Design review of the part built by this model. Coordinates are the model's own, in mm. Face numbers are marked on the shaded views. Coordinates: 2 decimals unless noted, no trailing zeros. Loops run counter-clockwise (first coordinate to the right, second up) from the corner with the lowest first, then second, coordinate; pieces in that order, holes last. Notation, with made-up numbers: (88, -18) - (110, -18) arc R18 cw to (110, 0) - close; hole circle Ø11 at (0, 7.5). An arc over 180 degrees is marked (long way). Answer in a Markdown table with one row per item. Add a question column.
(1) We need section A-A, the plane x = 3.8. Write out the cut boundary in (y, z).
(2) Clearance check with flat-ended pins moving along their axes: pin 1 (12 mm diameter, centred on y = -18, z = 90, fed in from +X); pin 2 (5 mm diameter, centred on y = -19.5, z = 28, fed in from +X); pin 3 (5 mm diameter, centred on x = 12.5, z = 86.5, fed in from -Y). State where each tip first meets the part, or that it passes through.
(3) We need section D-D, the plane x = 59.9. Write out the cut boundary in (y, z), plus the area to 3 significant figures.
(4) To check wall thickness, follow L1, parallel to Z at x = 116, y = -1.8; L2, parallel to X at y = -1.65, z = 115.9; L3, parallel to X at y = -2, z = 27. State the ranges of each line that lie inside material, in increasing order. Write a range as [from, to].
(5) We need section C-C, the plane z = 59.8. Write out the cut boundary in (x, y), plus the area to 3 significant figures.
(6) We need section B-B, the plane z = 3.7. Write out the cut boundary in (x, y), plus the area to 3 significant figures.
(7) The part is to be moulded in two halves that separate along X. For the marked faces 1 and 2, say which applies: released by +X, released by -X, zero draft, split by the parting line, or undercut.
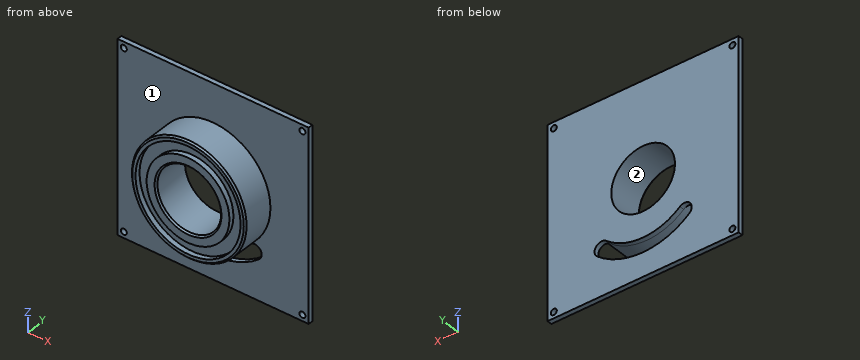
from build123d import *

# Parameters (mm, degrees)
SKETCH054_W     = 120
SKETCH054_H     = 120
PAD015_DEPTH    = 3
SKETCH065_R     = 1.9
POCKET034_DEPTH = 3.001
SKETCH064_R     = 20
POCKET036_DEPTH = 3.001
SKETCH058_R     = 36
PAD013_DEPTH    = 20
SKETCH055_R     = 20
POCKET035_DEPTH = 20.001
SKETCH056_R     = 33
SKETCH056_R_2   = 26
POCKET037_DEPTH = 3.2
CHAMFER003_SIZE = 1
CHAMFER002_SIZE = 1
POCKET042_DEPTH = 3.001


with BuildPart() as part:
    # Sketch054 → Pad015 (new body)
    with BuildSketch(Plane.XZ):
        with Locations((60, 60)):
            Rectangle(SKETCH054_W, SKETCH054_H)
    extrude(amount=PAD015_DEPTH)

    # Sketch065 (on Face6 of Pad015) → Pocket034 (cut, through all)
    with BuildSketch(Plane.XZ.offset(3)):
        with Locations((3.9, 3.9)):
            Circle(SKETCH065_R)
        with Locations((116.1, 3.9)):
            Circle(SKETCH065_R)
        with Locations((116.1, 116.1)):
            Circle(SKETCH065_R)
        with Locations((3.9, 116.1)):
            Circle(SKETCH065_R)
    extrude(amount=-POCKET034_DEPTH, mode=Mode.SUBTRACT)

    # Sketch064 (on Face5 of Pocket034) → Pocket036 (cut, through all)
    with BuildSketch(Plane.XZ.offset(3)):
        with Locations((60, 60)):
            Circle(SKETCH064_R)
    extrude(amount=-POCKET036_DEPTH, mode=Mode.SUBTRACT)

    # Sketch058 (on Face5 of Pocket036) → Pad013 (join)
    with BuildSketch(Plane.XZ.offset(3)):
        with Locations((60, 60)):
            Circle(SKETCH058_R)
    extrude(amount=PAD013_DEPTH)

    # Sketch055 (on Face13 of Pad013) → Pocket035 (cut, through all)
    with BuildSketch(Plane(origin=(0, -3, 0), x_dir=(1, 0, 0), z_dir=(0, 1, 0))):
        with Locations((60, -60)):
            Circle(SKETCH055_R)
    extrude(amount=-POCKET035_DEPTH, mode=Mode.SUBTRACT)

    # Sketch056 (on Face14 of Pocket035) → Pocket037 (cut)
    with BuildSketch(Plane.XZ.offset(23)):
        with Locations((60, 60)):
            Circle(SKETCH056_R)
        with Locations((60, 60)):
            Circle(SKETCH056_R_2, mode=Mode.SUBTRACT)
    extrude(amount=-POCKET037_DEPTH, mode=Mode.SUBTRACT)

    # Chamfer003
    chamfer003_edges = [part.edges().sort_by_distance(p)[0] for p in [
        (40, -23, 60),
    ]]
    chamfer(chamfer003_edges, length=CHAMFER003_SIZE)

    # Chamfer002
    chamfer002_edges = [part.edges().sort_by_distance(p)[0] for p in [
        (24, -23, 60),
    ]]
    chamfer(chamfer002_edges, length=CHAMFER002_SIZE)

    # Sketch066 (on Face3 of Chamfer002) → Pocket042 (cut, through all)
    with BuildSketch(Plane.XZ.offset(3)):
        with BuildLine():
            ThreePointArc((36.859646, 32.4224), (60, 24), (83.140354, 32.4224))
            ThreePointArc((88.925456, 25.528011), (89.480105, 31.867761), (83.140354, 32.4224))
            ThreePointArc((31.074571, 25.527989), (60.000017, 15), (88.925456, 25.528011))
            ThreePointArc((36.859646, 32.4224), (30.519908, 31.867728), (31.074571, 25.527989))
        make_face()
    extrude(amount=-POCKET042_DEPTH, mode=Mode.SUBTRACT)


with BuildPart() as part_1:
    # Body007 placement: moved
    add(part.part.moved(Location((-0.1, 0.5, -0.2))))


solid = part_1.part
Responses:
| question | item | result |
|---|---|---|
| 1 | outline | (-2.5, -0.2) - (0.5, -0.2) - (0.5, 1.8) - (-2.5, 1.8) - close; (-2.5, 5.6) - (0.5, 5.6) - (0.5, 114) - (-2.5, 114) - close; (-2.5, 117.8) - (0.5, 117.8) - (0.5, 119.8) - (-2.5, 119.8) - close |
| 2 | pin 1 | stops at x = 86.55 |
| 2 | pin 2 | stops at x = 80.82 |
| 2 | pin 3 | stops at y = -2.5 |
| 3 | outline | (-22.5, 24.8) - (-21.5, 23.8) - (0.5, 23.8) - (0.5, 39.8) - (-21.5, 39.8) - (-22.5, 38.8) - (-22.5, 33.8) - (-19.3, 33.8) - (-19.3, 26.8) - (-22.5, 26.8) - close; (-22.5, 80.8) - (-21.5, 79.8) - (0.5, 79.8) - (0.5, 119.8) - (-2.5, 119.8) - (-2.5, 95.8) - (-21.5, 95.8) - (-22.5, 94.8) - (-22.5, 92.8) - (-19.3, 92.8) - (-19.3, 85.8) - (-22.5, 85.8) - close; (-2.5, -0.2) - (0.5, -0.2) - (0.5, 14.8) - (-2.5, 14.8) - close |
| 3 | area | 806 mm2 |
| 4 | L1 | z = [-0.2, 1.8], [5.6, 114], [117.8, 119.8] |
| 4 | L2 | x = [-0.1, 1.9], [5.7, 114.1], [117.9, 119.9] |
| 4 | L3 | x = [-0.1, 29.73], [45.06, 74.74], [90.07, 119.9] |
| 5 | outline | (-0.1, -2.5) - (23.9, -2.5) - (23.9, -21.5) - (24.9, -22.5) - (26.9, -22.5) - (26.9, -19.3) - (33.9, -19.3) - (33.9, -22.5) - (38.9, -22.5) - (39.9, -21.5) - (39.9, 0.5) - (-0.1, 0.5) - close; (79.9, -21.5) - (80.9, -22.5) - (85.9, -22.5) - (85.9, -19.3) - (92.9, -19.3) - (92.9, -22.5) - (94.9, -22.5) - (95.9, -21.5) - (95.9, -2.5) - (119.9, -2.5) - (119.9, 0.5) - (79.9, 0.5) - close |
| 5 | area | 833 mm2 |
| 6 | outline | (-0.1, -2.5) - (1.9, -2.5) - (1.9, 0.5) - (-0.1, 0.5) - close; (5.7, -2.5) - (114.1, -2.5) - (114.1, 0.5) - (5.7, 0.5) - close; (117.9, -2.5) - (119.9, -2.5) - (119.9, 0.5) - (117.9, 0.5) - close |
| 6 | area | 337 mm2 |
| 7 | face 1 | zero draft |
| 7 | face 2 | undercut |
